```python
from build123d import *

# Parameters (mm, degrees)
SKETCH1_W           = 240
SKETCH1_H           = 126.92
BOSS_EXTRUDE1_DEPTH = 10
CHAMFER1_SIZE2      = 27.474774195
CHAMFER1_SIZE       = 10
CHAMFER3_SIZE2      = 10
CHAMFER3_SIZE       = 3.639702343


with BuildPart() as part:
    # Sketch1 → Boss-Extrude1 (new body)
    with BuildSketch(Plane(origin=(0, 0, 0), x_dir=(1, 0, 0), z_dir=(0, 1, 0))):
        with Locations((120, 63.46)):
            Rectangle(SKETCH1_W, SKETCH1_H)
    extrude(amount=BOSS_EXTRUDE1_DEPTH)

    # Chamfer1
    chamfer1_edges = [part.edges().sort_by_distance(p)[0] for p in [
        (120, 10, -126.92),
    ]]
    chamfer1_side = [part.faces().sort_by_distance(p)[0] for p in [
        (120, 9.8, -126.92),
    ]]
    chamfer(chamfer1_edges, length=CHAMFER1_SIZE - 0.0001, length2=CHAMFER1_SIZE2 - 0.0001, reference=chamfer1_side[0])  # a hair under: the kernel refuses the full size

    # Chamfer3
    chamfer3_edges = [part.edges().sort_by_distance(p)[0] for p in [
        (120, 10, 0),
    ]]
    chamfer3_side = [part.faces().sort_by_distance(p)[0] for p in [
        (120, 10, -0.072794047),
    ]]
    chamfer(chamfer3_edges, length=CHAMFER3_SIZE - 0.0001, length2=CHAMFER3_SIZE2 - 0.0001, reference=chamfer3_side[0])  # a hair under: the kernel refuses the full size


solid = part.part
```
Design review of the part built by this model. Coordinates are the model's own, in mm. Coordinates: 2 decimals unless noted, no trailing zeros. Order: outer loops, then holes, each group sorted by start corner. A loop starts at its lowest first (then second) coordinate and runs counter-clockwise, first axis right, second up.
1) Wall thickness on line 1 along Y through (x, z) = (224, -109); line 2 along Y through (x, z) = (136.5, -104): over which ranges is each line inside the solid? List them lowest first.
2) Clearance check with flat-ended pins moving along their axes: pin 1 (5 mm diameter, centred on x = 174.5, z = -85, fed in from -Y); pin 2 (4 mm diameter, centred on x = 125.5, y = 8, fed in from +Z). State where each tip first meets the part, or that it passes through.
3) Take a section at B-B, the plane y = 3.5. Give the boundary of the cut face in (x, z), and give its area (3 significant figures).
Returned:
1. line 1: y = 0 to 6.52
1. line 2: y = 0 to 8.34
2. pin 1: stops at y = 0
2. pin 2: stops at z = -2.18
3. outline: (0, -117.3) - (240, -117.3) - (240, -1.27) - (0, -1.27) - close
3. area: 27,800 mm2
